Autodesk Inventor part; units mm, degrees
ref_plane "YZ Plane" through (0, 0, 0) normal (1, 0, 0) x (0, 1, 0)
ref_plane "XZ Plane" through (0, 0, 0) normal (0, 1, 0) x (-1, 0, 0)
ref_plane "XY Plane" through (0, 0, 0) normal (0, 0, 1) x (1, 0, 0)
sketch "Boceto1" plane through (0, 0, 0) normal (0, 0, 1) x (1, 0, 0)
  line L0 (-35, 37.5) -> (35, 37.5)
  line L1 (35, 37.5) -> (35, -37.5)
  line L2 (35, -37.5) -> (-35, -37.5)
  line L3 (-35, -37.5) -> (-35, 37.5)
  point P0 (0, 0)
  point P1 (-35, 0)
  point P2 (0, 37.5)
  dimension "d0" = 70
  dimension "d1" = 75
extrude "Extrusión1" add sketch "Boceto1" along normal blind 1
sketch "Boceto2" plane through (0, 0, 1) normal (0, 0, 1) x (1, 0, 0)
  line L0 (-27, -27) -> (-15, -27)
  line L1 (-15, -27) -> (-15, -15)
  line L2 (-15, -15) -> (-27, -15)
  line L3 (-27, -15) -> (-27, -27)
  line L4 (-13, -27) -> (-1, -27)
  line L5 (-1, -27) -> (-1, -15)
  line L6 (-1, -15) -> (-13, -15)
  line L7 (-13, -15) -> (-13, -27)
  line L8 (1, -27) -> (13, -27)
  line L9 (13, -27) -> (13, -15)
  line L10 (13, -15) -> (1, -15)
  line L11 (1, -15) -> (1, -27)
  line L12 (15, -27) -> (27, -27)
  line L13 (27, -27) -> (27, -15)
  line L14 (27, -15) -> (15, -15)
  line L15 (15, -15) -> (15, -27)
  line L16 (-27, -13) -> (-15, -13)
  line L17 (-15, -13) -> (-15, -1)
  line L18 (-15, -1) -> (-27, -1)
  line L19 (-27, -1) -> (-27, -13)
  line L20 (-13, -13) -> (-1, -13)
  line L21 (-1, -13) -> (-1, -1)
  line L22 (-1, -1) -> (-13, -1)
  line L23 (-13, -1) -> (-13, -13)
  line L24 (1, -13) -> (13, -13)
  line L25 (13, -13) -> (13, -1)
  line L26 (13, -1) -> (1, -1)
  line L27 (1, -1) -> (1, -13)
  line L28 (15, -13) -> (27, -13)
  line L29 (27, -13) -> (27, -1)
  line L30 (27, -1) -> (15, -1)
  line L31 (15, -1) -> (15, -13)
  line L32 (-27, 1) -> (-15, 1)
  line L33 (-15, 1) -> (-15, 13)
  line L34 (-15, 13) -> (-27, 13)
  line L35 (-27, 13) -> (-27, 1)
  line L36 (-13, 1) -> (-1, 1)
  line L37 (-1, 1) -> (-1, 13)
  line L38 (-1, 13) -> (-13, 13)
  line L39 (-13, 13) -> (-13, 1)
  line L40 (1, 1) -> (13, 1)
  line L41 (13, 1) -> (13, 13)
  line L42 (13, 13) -> (1, 13)
  line L43 (1, 13) -> (1, 1)
  line L44 (15, 1) -> (27, 1)
  line L45 (27, 1) -> (27, 13)
  line L46 (27, 13) -> (15, 13)
  line L47 (15, 13) -> (15, 1)
  line L48 (-27, 15) -> (-15, 15)
  line L49 (-15, 15) -> (-15, 27)
  line L50 (-15, 27) -> (-27, 27)
  line L51 (-27, 27) -> (-27, 15)
  line L52 (-13, 15) -> (-1, 15)
  line L53 (-1, 15) -> (-1, 27)
  line L54 (-1, 27) -> (-13, 27)
  line L55 (-13, 27) -> (-13, 15)
  line L56 (1, 15) -> (13, 15)
  line L57 (13, 15) -> (13, 27)
  line L58 (13, 27) -> (1, 27)
  line L59 (1, 27) -> (1, 15)
  line L60 (15, 15) -> (27, 15)
  line L61 (27, 15) -> (27, 27)
  line L62 (27, 27) -> (15, 27)
  line L63 (15, 27) -> (15, 15)
  line L64 (-1, -1) -> (1, 1) construction
  point P0 (0, 0)
  point P1 (0, 0)
  dimension "d6" = 14
  dimension "d9" = 14
  dimension "d12" = 12
extrude "Extrusión2" add sketch "Boceto2" along normal blind 0.1
equation "\"d9\" = d6"
properties part number "botonera"
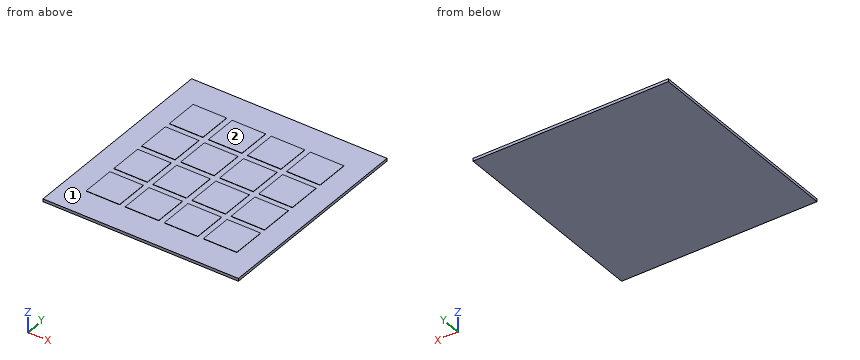
For this review, take the finished solid that the model builds, in its own axes (mm). Face numbers are marked on the shaded views. A direction names the side the tool comes from. Give positions to 0.01 mm unless a question says otherwise; leave off trailing zeros. Loops run counter-clockwise (first coordinate to the right, second up) from the corner with the lowest first, then second, coordinate; pieces in that order, holes last. Notation, with made-up numbers: M 69,43.25 L 91,43.25 A13 ccw 91,60.25 Z; hole C 53.5,86.5 d11. An arc over 180 degrees is marked long. Put each result on its own line as item: value. Start each with the question number.
(1) Add section B-B, the plane y = -6. Write out the cut boundary in (x, z).
(2) Wall thickness on L1, parallel to Y at x = 24.5, z = 1.05; L2, parallel to Z at x = 29, y = 1.5: over which ranges is each line inside the solid? List them lowest first.
(3) Machinability: for the marked faces 1 and 2, which of the approach directions +Z, -Z, +X, -X, +Y, -Y give a long, thin tool a straight path to every point of the face, cutting with its end or side? Answer none if there is none.
(4) Add section A-A, the plane x = 12. Write out the cut boundary in (y, z).
Result:
1. outline: M -35,0 L 35,0 L 35,1 L 27,1 L 27,1.1 L 15,1.1 L 15,1 L 13,1 L 13,1.1 L 1,1.1 L 1,1 L -1,1 L -1,1.1 L -13,1.1 L -13,1 L -15,1 L -15,1.1 L -27,1.1 L -27,1 L -35,1 Z
2. L1: y = -27 to -15, -13 to -1, 1 to 13, 15 to 27
2. L2: z = 0 to 1
3. face 1: +Z
3. face 2: +Z, +X, -X, +Y, -Y
4. outline: M -37.5,0 L 37.5,0 L 37.5,1 L 27,1 L 27,1.1 L 15,1.1 L 15,1 L 13,1 L 13,1.1 L 1,1.1 L 1,1 L -1,1 L -1,1.1 L -13,1.1 L -13,1 L -15,1 L -15,1.1 L -27,1.1 L -27,1 L -37.5,1 Z
